Verification items for the finished model (mm, model axes). Give positions to 0.01 mm unless a question says otherwise; leave off trailing zeros. Order: outer loops, then holes, each group sorted by start corner. A loop starts at its lowest first (then second) coordinate and runs counter-clockwise, first axis right, second up. Notation, with made-up numbers: (51.25, 21) -> (55.25, 21) arc R19 cw to (55.25, 50) -> close; hole circle Ø1 at (35.25, 88). An arc over 180 degrees is marked (long way). One line per question, with ' | ' between items. Start each with the question number.
Q1. Go/stop test with a flat-tipped pin: pin 1 (1.5 mm diameter, centred on x = -2, z = -1, fed in from +Y). Record where the tip stops, or that it passes through.
Q2. Section check A-A on y = -0.5. Record the cut outline in (x, z) (1 decimal), plus the area to 3 significant figures.
Q3. Section check C-C on x = 0. Record the cut outline in (y, z), plus the area to 3 significant figures.
Q4. Section check B-B on z = 0. Record the cut outline in (x, y).
Q5. Material ranges on probe 1 along Z at (x, y) = (-0.75, -0.25); probe 2 along Z at (x, y) = (2, -0.1); probe 3 along Z at (x, y) = (2.5, -0.15), recorded low to high. Write a range as [from, to].
Q6. Section check D-D on z = 1. Give the number of separate pieces and of enclosed holes in the cut face, plus the area to 3 significant figures.
Q7. Mould release check, pull along Z, two halves, no side actions. Record for faces 1 (the cylindrical face through (-0.455, -0.44, 3.463)), 2 (the flat face through (1, 0, 0)), 3 (the cylindrical face through (1.6, -0.438, -1.044)): released by +Z, released by -Z, zero draft, split by the parting line, or undercut.
from build123d import *

# Parameters (mm, degrees)
F0_R     = 3.4925
F0_R_2   = 0.2794
F1_DEPTH = 0.889
F2_SIZE  = 0.127


with BuildPart() as f1:
    # F0 (on Front) → F1 (new body)
    with BuildSketch(Plane.XZ):
        Circle(F0_R)
        with BuildLine():
            ThreePointArc((0.541666, -1.403826), (-0.582476, -1.692408), (-1.732036, -1.532768))
            ThreePointArc((-1.732036, -1.532768), (-1.70195, -0.854412), (-1.490076, -0.209291))
            ThreePointArc((-1.490076, -0.209291), (-0.762626, -1.297124), (0.541666, -1.403826))
        make_face(mode=Mode.SUBTRACT)
        Circle(F0_R_2, mode=Mode.SUBTRACT)
        with BuildLine():
            ThreePointArc((0.944916, 1.17101), (1.756906, 0.341765), (2.193434, -0.733604))
            ThreePointArc((2.193434, -0.733604), (1.590918, -1.046726), (0.92629, -1.185799))
            ThreePointArc((0.92629, -1.185799), (1.504656, -0.011892), (0.944916, 1.17101))
        make_face(mode=Mode.SUBTRACT)
        with BuildLine():
            ThreePointArc((-0.461398, 2.266371), (0.111032, 1.901138), (0.563787, 1.39509))
            ThreePointArc((0.563787, 1.39509), (-0.742029, 1.309016), (-1.486582, 0.232816))
            ThreePointArc((-1.486582, 0.232816), (-1.17443, 1.350643), (-0.461398, 2.266371))
        make_face(mode=Mode.SUBTRACT)
    extrude(amount=F1_DEPTH)

    # F2
    f2_edges = [f1.edges().sort_by_distance(p)[0] for p in [
        (-3.4925, -0.889, 0),
        (-3.4925, 0, 0),
    ]]
    chamfer(f2_edges, length=F2_SIZE)


solid = f1.part
Filled in:
1) pin 1: y = 0
2) outline: circle Ø7 at (0, 0); hole (-1.7, -1.5) arc R3 ccw to (0.5, -1.4) arc R1.5 cw to (-1.5, -0.2) arc R2.5 ccw to start; hole (-1.5, 0.2) arc R1.5 cw to (0.6, 1.4) arc R2.5 ccw to (-0.5, 2.3) arc R3 ccw to start; hole circle Ø0.6 at (0, 0); hole (0.9, -1.2) arc R2.5 ccw to (2.2, -0.7) arc R3 ccw to (0.9, 1.2) arc R1.5 cw to start | area: 35.1 mm²
3) outline: (-0.89, -3.37) -> (-0.76, -3.49) -> (-0.13, -3.49) -> (0, -3.37) -> (0, -1.6) -> (-0.89, -1.6) -> close; (-0.89, -1.5) -> (0, -1.5) -> (0, -0.28) -> (-0.89, -0.28) -> close; (-0.89, 0.28) -> (0, 0.28) -> (0, 1.5) -> (-0.89, 1.5) -> close; (-0.89, 1.99) -> (0, 1.99) -> (0, 3.37) -> (-0.13, 3.49) -> (-0.76, 3.49) -> (-0.89, 3.37) -> close | area: 5.16 mm²
4) outline: (-3.49, -0.76) -> (-3.37, -0.89) -> (-0.28, -0.89) -> (-0.28, 0) -> (-3.37, 0) -> (-3.49, -0.13) -> close; (0.28, -0.89) -> (1.5, -0.89) -> (1.5, 0) -> (0.28, 0) -> close; (1.95, -0.89) -> (3.37, -0.89) -> (3.49, -0.76) -> (3.49, -0.13) -> (3.37, 0) -> (1.95, 0) -> close
5) probe 1: [-3.41, -1.7], [-1.3, 1.3], [1.98, 3.41] | probe 2: [-2.83, -0.86], [-0.11, 2.83] | probe 3: [-2.44, 2.44]
6) separate pieces: 3 | enclosed holes: 0 | area: 5.70 mm²
7) face 1: split by the parting line | face 2: zero draft | face 3: undercut
